For this review, take the finished solid that the model builds, in its own axes (mm). Face numbers are marked on the shaded views. A direction names the side the tool comes from. Coordinates: 2 decimals unless noted, no trailing zeros. Order: outer loops, then holes, each group sorted by start corner. A loop starts at its lowest first (then second) coordinate and runs counter-clockwise, first axis right, second up. Notation, with made-up numbers: (14.25, 66.25) -> (48.25, 66.25) arc R16 cw to (48.25, 81.25) -> close; hole circle Ø1 at (69, 15.5). An arc over 180 degrees is marked (long way). Return JSON: item names as keys, results as strings. Group by question number.
Item 1: For line 1 along X through (y, z) = (160.5, -116); line 2 along Y through (x, z) = (-52.5, -34), list the stretches that pass through material, from the lowest coordinate up.
Item 2: Insertion check: pin 1 (5 mm diameter, centred on x = -44, y = 177, fed in from -Z). The pin has a flat end and moves straight along its axis. Give the tip position at first contact, or say it passes through.
Item 3: Take a section at C-C (z = -114.5). Write out the cut boundary in (x, y), then the cut area to 3 significant figures.
Item 4: Take a section at A-A (x = -45). Write out the cut boundary in (y, z).
Item 5: Machinability: for the marked faces 5 and 6, which of the approach directions +Z, -Z, +X, -X, +Y, -Y give a long, thin tool a straight path to every point of the face, cutting with its end or side? Answer none if there is none.
Item 6: Take a section at B-B (y = 166). Write out the cut boundary in (x, z), then the cut area to 3 significant figures.
Item 7: Draft analysis for pull direction Y (two halves, no side actions). For the marked faces 1, 2, 3 and 4, state which applies: +Y half, -Y half, draft (parallel to the pull), parting line (faces both ways), or undercut.
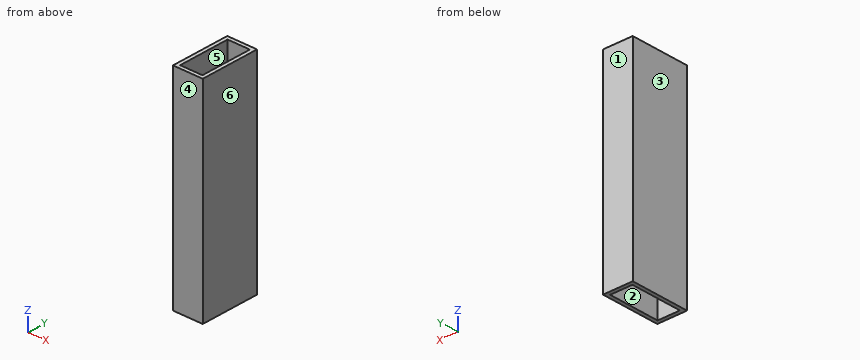
Autodesk Inventor part; units mm, degrees
ref_plane "YZ Plane" through (0, 0, 0) normal (1, 0, 0) x (0, 1, 0)
ref_plane "XZ Plane" through (0, 0, 0) normal (0, 1, 0) x (-1, 0, 0)
ref_plane "XY Plane" through (0, 0, 0) normal (0, 0, 1) x (1, 0, 0)
sketch "Sketch1" plane through (0, 0, 0) normal (0, 0, 1) x (1, 0, 0)
  line L0 (-61.9417, 182.4966) -> (-36.5417, 182.4966)
  line L1 (-36.5417, 182.4966) -> (-36.5417, 131.6966)
  line L2 (-36.5417, 131.6966) -> (-61.9417, 131.6966)
  line L3 (-61.9417, 131.6966) -> (-61.9417, 182.4966)
  line L4 (-58.7667, 179.3216) -> (-39.7167, 179.3216)
  line L5 (-39.7167, 179.3216) -> (-39.7167, 134.8716)
  line L6 (-39.7167, 134.8716) -> (-58.7667, 134.8716)
  line L7 (-58.7667, 134.8716) -> (-58.7667, 179.3216)
  point P0 (0, 0)
  dimension "d0" = 25.4
  dimension "d1" = 50.8
  dimension "d2" = 3.175
extrude "Extrusion1" add sketch "Sketch1" against normal blind 177.8
properties part number "Motor Mount 2"
Findings below:
{
 "1": {"line 1": "x = -61.94 to -58.77, -39.72 to -36.54", "line 2": "y = 131.7 to 134.87, 179.32 to 182.5"},
 "2": {"pin 1": "stops at z = -177.8"},
 "3": {"outline": "(-61.94, 131.7) -> (-36.54, 131.7) -> (-36.54, 182.5) -> (-61.94, 182.5) -> close; hole (-58.77, 134.87) -> (-39.72, 134.87) -> (-39.72, 179.32) -> (-58.77, 179.32) -> close", "area": "444 mm2"},
 "4": {"outline": "(131.7, -177.8) -> (134.87, -177.8) -> (134.87, 0) -> (131.7, 0) -> close; (179.32, -177.8) -> (182.5, -177.8) -> (182.5, 0) -> (179.32, 0) -> close"},
 "5": {"face 5": "+Z, -Z", "face 6": "+Z, -Z, +X, +Y, -Y"},
 "6": {"outline": "(-61.94, -177.8) -> (-58.77, -177.8) -> (-58.77, 0) -> (-61.94, 0) -> close; (-39.72, -177.8) -> (-36.54, -177.8) -> (-36.54, 0) -> (-39.72, 0) -> close", "area": "1,130 mm2"},
 "7": {"face 1": "+Y half", "face 2": "undercut", "face 3": "draft", "face 4": "-Y half"}
}
